Autodesk Inventor part; units mm, degrees
ref_plane "YZ Plane" through (0, 0, 0) normal (1, 0, 0) x (0, 1, 0)
ref_plane "XZ Plane" through (0, 0, 0) normal (0, 1, 0) x (-1, 0, 0)
ref_plane "XY Plane" through (0, 0, 0) normal (0, 0, 1) x (1, 0, 0)
sketch "Sketch1" plane through (0, 0, 0) normal (0, 1, 0) x (-1, 0, 0)
  point P0 (0, 0)
sketch "Sketch2" plane through (0, 0, 0) normal (0, 1, 0) x (-1, 0, 0)
  line L0 (0, 0) -> (-132, 0)
  line L1 (-132, 0) -> (-132, -20)
  line L2 (-132, -20) -> (0, -20)
  line L3 (0, -20) -> (0, 0)
  dimension "d0" = 132
  dimension "d1" = 20
extrude "Extrusion1" add sketch "Sketch2" along normal blind 3
sketch "Sketch3" plane through (0, 3, 0) normal (0, 1, 0) x (1, 0, 0)
  line L0 (132, 20) -> (0, 20)
  line L1 (0, 20) -> (15, 20)
  line L2 (15, 20) -> (15, 32)
  line L3 (15, 32) -> (0, 32)
  line L4 (0, 32) -> (0, 20)
  line L5 (3, 29) -> (12, 29)
  line L6 (12, 29) -> (12, 26)
  line L7 (12, 26) -> (3, 26)
  line L8 (3, 26) -> (3, 29)
  line L9 (132, 0) -> (132, 20)
  line L10 (112, 20) -> (97, 20)
  line L11 (97, 20) -> (97, 32)
  line L12 (97, 32) -> (112, 32)
  line L13 (112, 32) -> (112, 20)
  line L14 (109, 29) -> (100, 29)
  line L15 (100, 29) -> (100, 26)
  line L16 (100, 26) -> (109, 26)
  line L17 (109, 26) -> (109, 29)
  point P0 (0, 0)
  dimension "d4" = 15
  dimension "d8" = 3
  dimension "d9" = 3
  dimension "d10" = 3
  dimension "d11" = 6
  dimension "d12" = 3
  dimension "d13" = 15
  dimension "d14" = 3
  dimension "d15" = 3
  dimension "d16" = 3
  dimension "d17" = 3
  dimension "d18" = 6
  dimension "d19" = 82
extrude "Extrusion2" add sketch "Sketch3" against normal blind 3
equation "\"d9\" = d8"
equation "\"d10\" = d8"
equation "\"d16\" = d15"
equation "\"d17\" = d15"
properties part number "ball-reload-right"
The model under review builds one solid part; all positions refer to its coordinate system, in mm. A direction names the side the tool comes from. Coordinates: 2 decimals unless noted, no trailing zeros. Loops run counter-clockwise (first coordinate to the right, second up) from the corner with the lowest first, then second, coordinate; pieces in that order, holes last.
(1) Draft analysis for pull direction X (two halves, no side actions). For faces 1 (the flat face through (104, 2, -32)), 2 (the flat face through (8, 2, -26)), 3 (the flat face through (132, 1, -10)), 4 (the flat face through (104, 2, -26)), state which applies: +X half, -X half, draft (parallel to the pull), parting line (faces both ways), or undercut.
Determined:
face 1: draft
face 2: undercut
face 3: +X half
face 4: undercut
(2) Wall thickness on L1, parallel to Z at x = 101.5, y = 0.45; L2, parallel to Z at x = 29, y = 2.9: over which ranges is each line inside the solid? List them lowest first.
Determined:
L1: z = -32 to -29, -26 to 0
L2: z = -20 to 0
(3) Tool access review of faces 5 (the flat face through (65, 1, 0)), 6 (the flat face through (15, 2, -26)), 7 (the flat face through (122, 1, -20)), 8 (the flat face through (3, 2, -27)), 9 (the flat face through (67, 3, -12)): name each direction out of +Z, -Z, +X, -X, +Y, -Y from which nothing blocks a thin tool from reaching the whole face with its end or side.
Determined:
face 5: +Z, +X, -X, +Y, -Y
face 6: -Z, +Y, -Y
face 7: -Z, +X, +Y, -Y
face 8: +Y, -Y
face 9: +Z, -Z, +X, -X, +Y
(4) Insertion check: P1, Ø0.9, axis at y = 1.5, z = -27, coming from the +X side; P2, Ø0.9, axis at x = 106.5, y = 1, coming from the +Z side. Each pin has a flat end and moves straight along its axis. Give the tip position at first contact, or say it passes through.
Determined:
P1: stops at x = 112
P2: stops at z = 0
(5) Consider section A-A, the plane z = -22.5. Give the boundary of the cut face in (x, y), plus the area to 3 significant figures.
Determined:
outline: (0, 0) - (15, 0) - (15, 3) - (0, 3) - close; (97, 0) - (112, 0) - (112, 3) - (97, 3) - close
area: 90.0 mm2
(6) Consider section B-B, the plane y = 2.2. Give the boundary of the cut face in (x, z).
Determined:
outline: (0, -32) - (15, -32) - (15, -20) - (97, -20) - (97, -32) - (112, -32) - (112, -20) - (132, -20) - (132, 0) - (0, 0) - close; hole (3, -29) - (12, -29) - (12, -26) - (3, -26) - close; hole (100, -29) - (109, -29) - (109, -26) - (100, -26) - close
(7) Consider section C-C, the plane x = 27. Give the boundary of the cut face in (y, z).
Determined:
outline: (0, -20) - (3, -20) - (3, 0) - (0, 0) - close
